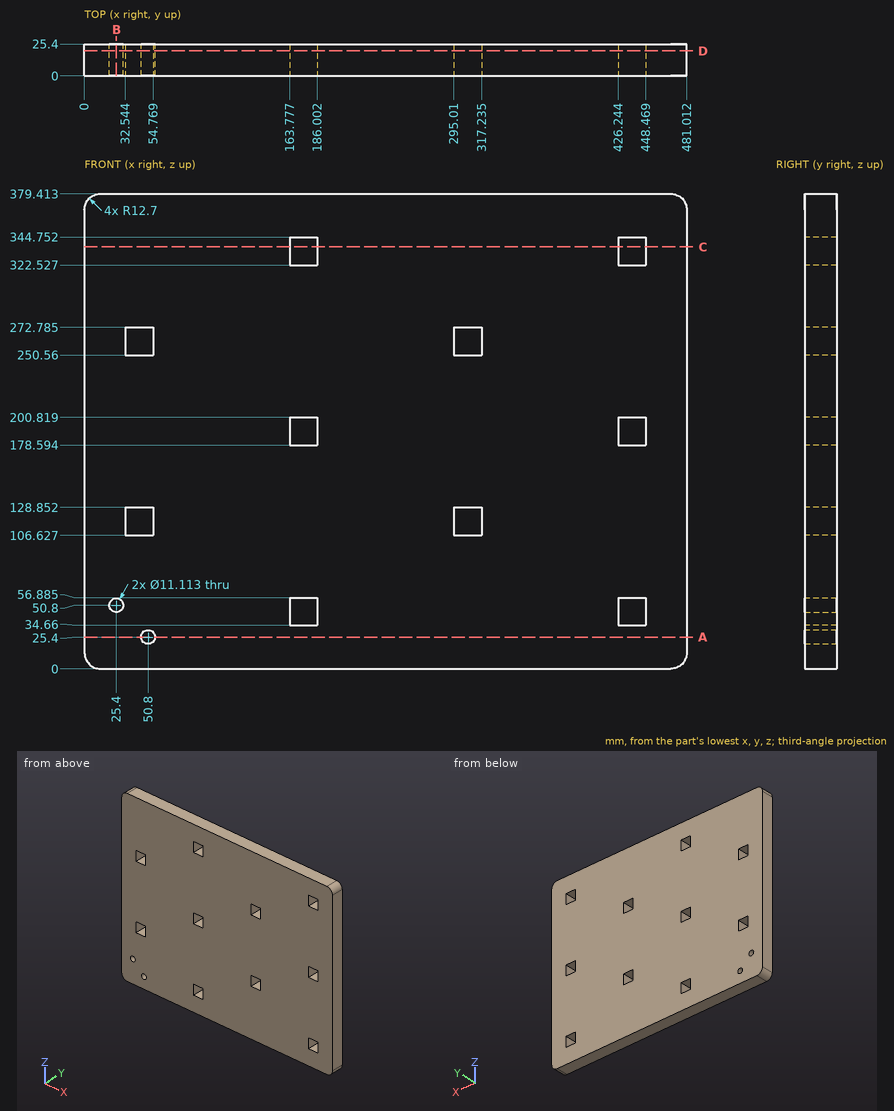
Print and shaded views of the part. All mm, measured from the part's lowest x, y and z. Give positions to 0.01 mm unless a question says otherwise; leave off trailing zeros. Write each loop counter-clockwise with the first axis right and the second up, starting at its lowest first coordinate (ties: lowest second). Pieces come first, ordered by that corner, then holes. Notation, with made-up numbers: (32, 11) -> (47, 11) arc R24 cw to (47, 34) -> close; hole circle Ø9 at (44.5, -38.5). An arc over 180 degrees is marked (long way). Use CSV: the item, a comma, the result in double quotes. Start each with the question number.
1) Cut at D-D on y = 20. Count the separate pieces of the cut face and the enclosed holes in it, plus the area to 3 significant figures.
2) Cut at C-C on z = 337. List the corners of the cut face in (x, y), plus the area to 3 significant figures.
3) Drill centre lines: L1, parallel to X at y = 17.75, z = 50.8; L2, parallel to Z at x = 44.5, y = 11.75 (1 decimal); L3, parallel to X at y = 12.5, z = 25.4. Where is each one in solid material? Low to high.
4) Cut at B-B on x = 25.4. List the corners of the cut face in (y, z).
5) Cut at A-A on z = 25.4. List the corners of the cut face in (x, y).
Final values:
1,separate pieces,"1"
1,enclosed holes,"12"
1,area,"177,000 mm2"
2,outline,"(0, 0) -> (163.78, 0) -> (163.78, 25.4) -> (0, 25.4) -> close; (186, 0) -> (426.24, 0) -> (426.24, 25.4) -> (186, 25.4) -> close; (448.47, 0) -> (481.01, 0) -> (481.01, 25.4) -> (448.47, 25.4) -> close"
2,area,"11,100 mm2"
3,L1,"x = 0 to 19.84, 30.96 to 163.78, 186 to 426.24, 448.47 to 481.01"
3,L2,"z = 0 to 106.6, 128.9 to 250.6, 272.8 to 379.4"
3,L3,"x = 0 to 45.24, 56.36 to 481.01"
4,outline,"(0, 0) -> (25.4, 0) -> (25.4, 45.24) -> (0, 45.24) -> close; (0, 56.36) -> (25.4, 56.36) -> (25.4, 379.41) -> (0, 379.41) -> close"
5,outline,"(0, 0) -> (45.24, 0) -> (45.24, 25.4) -> (0, 25.4) -> close; (56.36, 0) -> (481.01, 0) -> (481.01, 25.4) -> (56.36, 25.4) -> close"
